Work out the finished part from the listing and answer in its coordinate system (mm). A direction names the side the tool comes from. Give positions to 0.01 mm unless a question says otherwise; leave off trailing zeros. Order: outer loops, then holes, each group sorted by start corner. A loop starts at its lowest first (then second) coordinate and runs counter-clockwise, first axis right, second up. Notation, with made-up numbers: (63.5, 85) - (69.5, 85) arc R19 ccw to (69.5, 100) - close; hole circle Ø8 at (66.5, 11). An arc over 180 degrees is marked (long way). Put each result on its own line as item: value.
```python
from build123d import *

# Parameters (mm, degrees)
F0_W     = 127
F0_H     = 69.85
F1_DEPTH = 44.45
F3_DEPTH = 44.45
F5_DEPTH = 31.75


with BuildPart() as f1:
    # F0 (on Front) → F1 (new body)
    with BuildSketch(Plane.XZ):
        with Locations((1.307353, 14.007352)):
            Rectangle(F0_W, F0_H)
    extrude(amount=F1_DEPTH)

    # F2 (on face) → F3 (cut)
    with BuildSketch(Plane.XZ.offset(44.45)):
        Polygon((17.309353, 48.932352), (64.807353, 10.832352), (64.807353, 48.932352), align=None)
        Polygon((-62.192647, 48.932352), (-62.192647, 10.832352), (-14.694647, 48.932352), align=None)
    extrude(amount=-F3_DEPTH, mode=Mode.SUBTRACT)

    # F4 (on face) → F5 (cut)
    with BuildSketch(Plane.XZ.offset(44.45)):
        Polygon((64.807353, 10.832352), (17.309353, 48.932352), (17.309353, 34.708352), (-14.694647, 34.708352), (-14.694647, 48.932352), (-62.192647, 10.832352), (-62.192647, -20.917648), (-30.442647, -20.917648), (-30.442647, -8.217648), (-11.392647, 10.832352), (14.007353, 10.832352), (33.057353, -8.217648), (33.057353, -20.917648), (64.807353, -20.917648), align=None)
    extrude(amount=-F5_DEPTH, mode=Mode.SUBTRACT)


solid = f1.part
```
(1) Section D-D, the plane y = -11 is taken. Write down the section's boundary in (x, z), then the cut area to 3 significant figures.
Geometry check:
outline: (-62.19, -20.92) - (64.81, -20.92) - (64.81, 10.83) - (17.31, 48.93) - (-14.69, 48.93) - (-62.19, 10.83) - close
area: 7,060 mm²
(2) Section C-C, the plane x = 8 is taken. Write down the section's boundary in (y, z), then the cut area to 3 significant figures.
Geometry check:
outline: (-44.45, -20.92) - (0, -20.92) - (0, 48.93) - (-44.45, 48.93) - (-44.45, 34.71) - (-12.7, 34.71) - (-12.7, 10.83) - (-44.45, 10.83) - close
area: 2,350 mm²
(3) Section A-A, the plane y = -25.5 is taken. Write down the section's boundary in (x, z), then the cut area to 3 significant figures.
Geometry check:
outline: (-30.44, -20.92) - (33.06, -20.92) - (33.06, -8.22) - (14.01, 10.83) - (-11.39, 10.83) - (-30.44, -8.22) - close; (-14.69, 34.71) - (17.31, 34.71) - (17.31, 48.93) - (-14.69, 48.93) - close
area: 2,110 mm²
(4) Straight lines are drawn through the part: line 1 (Z direction, x = -2.5, y = -31); line 2 (Y direction, x = -51.5, z = 7); line 3 (X direction, y = -25, z = 45.5). For each, find the intervals that lie inside material, in ascending order.
Geometry check:
line 1: z = -20.92 to 10.83, 34.71 to 48.93
line 2: y = -12.7 to 0
line 3: x = -14.69 to 17.31
(5) Given pin 1 (10 mm diameter, centred on y = -20, z = 3.5, fed in from +X); pin 2 (3 mm diameter, centred on x = 31, y = -23, fed in from +Z); pin 3 (15.5 mm diameter, centred on y = -34.5, z = 39, fed in from +X); pin 4 (12 mm diameter, centred on x = -34, z = 26.5, fed in from +Y), each flat-ended and moving along its own axis, determine where each tip first touches the part or whether it passes through.
Geometry check:
pin 1: stops at x = 26.34
pin 2: stops at z = -4.66
pin 3: stops at x = 17.31
pin 4: stops at y = 0
(6) Section B-B, the plane z = -16 is taken. Write down the section's boundary in (x, y), then the cut area to 3 significant figures.
Geometry check:
outline: (-62.19, -12.7) - (-30.44, -12.7) - (-30.44, -44.45) - (33.06, -44.45) - (33.06, -12.7) - (64.81, -12.7) - (64.81, 0) - (-62.19, 0) - close
area: 3,630 mm²
(7) A tool of negligible diameter and unlimited length cuts with its end or side. For faces 5 (the face through (17.309, -29, 42)), 6 (the face through (-14.695, -29, 42)), 7 (the face through (23.4, -28.8, 1.44)), 8 (the face through (33.057, -29, -14)), from which of +Z, -Z, +X, -X, +Y, -Y can it reach the whole face along a straight path? Write none if from no direction.
Geometry check:
face 5: +Z, +X, -Y
face 6: +Z, -X, -Y
face 7: +X, -Y
face 8: +Z, -Z, +X, -Y
(8) Determine the mould class of faces 1 (the face through (1, -29, 10.832)), 2 (the face through (-30.443, -29, -15)), 3 (the face through (0, -17, -20.918)), 4 (the face through (2, -29, 34.708)) for opening direction Z: pulls with the +Z half, pulls with the -Z half, needs draft (parallel to the pull), parting line crosses it, or undercut.
Geometry check:
face 1: undercut
face 2: needs draft
face 3: pulls with the -Z half
face 4: undercut
